Design review of the part built by this model. Coordinates are the model's own, in mm. Face numbers are marked on the shaded views. A direction names the side the tool comes from. Coordinates: 2 decimals unless noted, no trailing zeros. Write each loop counter-clockwise with the first axis right and the second up, starting at its lowest first coordinate (ties: lowest second). Pieces come first, ordered by that corner, then holes.
Q1. Take a section at D-D (z = -3.5). Give the boundary of the cut face in (x, y), and give its area (3 significant figures).
Q2. Machinability: for the marked faces 5, 6 and 7, which of the approach directions +Z, -Z, +X, -X, +Y, -Y give a long, thin tool a straight path to every point of the face, cutting with its end or side? Answer none if there is none.
Q3. Take a section at A-A (x = 0). Give the boundary of the cut face in (y, z), and give its area (3 significant figures).
Q4. Mouldability with a two-part tool opening along Y and no side actions: class the marked faces 1, 2, 3 and 4 as pulls with the +Y half, pulls with the -Y half, needs draft (parallel to the pull), parting line crosses it, or undercut.
Q5. For probe 1 along Y at (x, z) = (0, 13); probe 2 along Z at (x, y) = (8.5, 1.5); probe 3 along Y at (x, z) = (-4.5, 12), list the stretches that pass through material, from the lowest coordinate up.
Q6. Take a section at B-B (y = -32). Give the boundary of the cut face in (x, z), and give its area (3 significant figures).
Q7. Take a section at C-C (z = 18.5). Give the boundary of the cut face in (x, y), and give its area (3 significant figures).
Q8. Insertion check: pin 1 (8 mm diameter, centred on x = 22, z = 13.5, fed in from +Y); pin 2 (2 mm diameter, centred on y = -56.5, z = 2.5, fed in from +X); pin 3 (7.5 mm diameter, centred on y = -59.5, z = 3, fed in from -X); pin 4 (2 mm diameter, centred on y = -57.5, z = 5, fed in from -X). Each pin has a flat end and moves straight along its axis. Give the tip position at first contact, or say it passes through.
```python
from build123d import *

# Parameters (mm, degrees)
SKETCH001_R   = 30
SKETCH001_R_2 = 18
PAD_DEPTH     = 30
PAD001_DEPTH  = 10
PAD002_DEPTH  = 7


with BuildPart() as part:
    # Sketch001 (on Sketch) → Pad (new body)
    with BuildSketch(Plane.XY):
        Circle(SKETCH001_R)
        Circle(SKETCH001_R_2, mode=Mode.SUBTRACT)
    extrude(amount=PAD_DEPTH)

    # Sketch002 (on Sketch) → Pad001 (join)
    with BuildSketch(Plane.XY):
        with BuildLine():
            ThreePointArc((30, 4.5e-05), (0, 30), (-30, 4.5e-05))
            Line((-30, 4.5e-05), (-30, -85))
            Line((30, -85), (-30, -85))
            Line((30, 4.5e-05), (30, -85))
        make_face()
    extrude(amount=-PAD001_DEPTH)

    # Sketch003 (on Sketch) → Pad002 (join)
    with BuildSketch(Plane.XY):
        with BuildLine():
            ThreePointArc((-15.008511, -25.975846), (-0.009828, -29.999998), (14.991489, -25.985674))
            Line((14.991489, -85), (14.991489, -25.985674))
            Line((14.991489, -85), (-15.008511, -85))
            Line((-15.008511, -25.975846), (-15.008511, -85))
        make_face()
        with BuildLine():
            ThreePointArc((7, -47.28644), (0, -40.28644), (-7, -47.28644))
            Line((-7, -47.28644), (-7, -67.28644))
            ThreePointArc((-7, -67.28644), (0, -74.28644), (7, -67.28644))
            Line((7, -47.28644), (7, -67.28644))
        make_face(mode=Mode.SUBTRACT)
    extrude(amount=PAD002_DEPTH)


solid = part.part
```
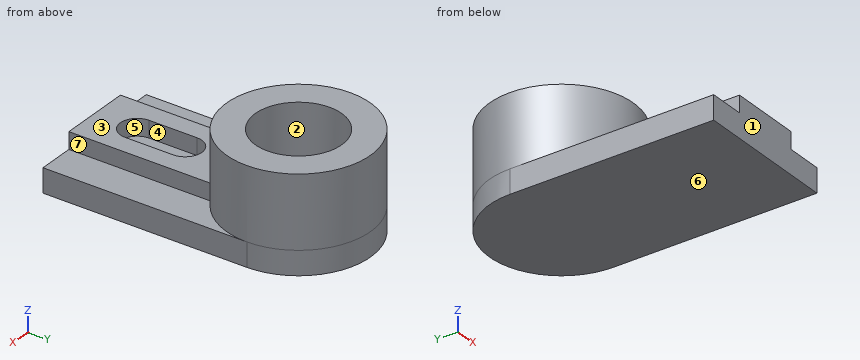
Response:
1. outline: (-30, -85) - (30, -85) - (30, 0) arc R30 ccw to (-30, 0) - close
1. area: 6,510 mm2
2. face 5: +Z
2. face 6: -Z, +X, -X, +Y, -Y
2. face 7: +Z, +X, -Y
3. outline: (-85, -10) - (30, -10) - (30, 30) - (18, 30) - (18, 0) - (-18, 0) - (-18, 30) - (-30, 30) - (-30, 7) - (-40.29, 7) - (-40.29, 0) - (-74.29, 0) - (-74.29, 7) - (-85, 7) - close
3. area: 2,020 mm2
4. face 1: pulls with the -Y half
4. face 2: undercut
4. face 3: needs draft
4. face 4: undercut
5. probe 1: y = -30 to -18, 18 to 30
5. probe 2: z = -10 to 0
5. probe 3: y = -29.66 to -17.43, 17.43 to 29.66
6. outline: (-30, -10) - (30, -10) - (30, 0) - (14.99, 0) - (14.99, 7) - (-15.01, 7) - (-15.01, 0) - (-30, 0) - close
6. area: 810 mm2
7. outline: circle Ø60 at (0, 0); hole circle Ø36 at (0, 0)
7. area: 1,810 mm2
8. pin 1: stops at y = 24
8. pin 2: stops at x = 14.99
8. pin 3: stops at x = -30
8. pin 4: stops at x = -15.01
